Check sheet for the modelled part. Datum: model origin and axes. Units: mm. Face numbers are marked on the shaded views. A direction names the side the tool comes from. Give positions to 0.01 mm unless a question says otherwise; leave off trailing zeros. Order: outer loops, then holes, each group sorted by start corner. A loop starts at its lowest first (then second) coordinate and runs counter-clockwise, first axis right, second up. Notation, with made-up numbers: (-17.5, 37.25) - (27.5, 37.25) arc R22 cw to (27.5, 46.25) - close; hole circle Ø3 at (38, -7.75). An arc over 180 degrees is marked (long way). Answer in a Markdown table with one row per item.
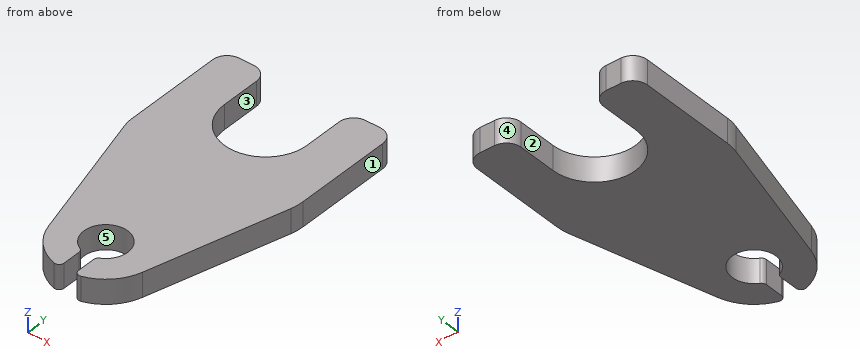
from build123d import *

# Parameters (mm, degrees)
BASE_EXTRUDE_DEPTH = 5


with BuildPart() as part:
    # Sketch1 → Base-Extrude (new body)
    with BuildSketch(Plane.XY):
        with BuildLine():
            Line((1.5, -4.898979486), (1.5, -8.645808233))
            ThreePointArc((1.5, -8.645808233), (1.899074787, -9.445113487), (2.777777778, -9.606453592))
            ThreePointArc((2.777777778, -9.606453592), (7.140306068, -7.001144853), (9.659258263, -2.588190451))
            Line((9.659258263, -2.588190451), (17.159258263, 25.402190606))
            ThreePointArc((17.159258263, 25.402190606), (17.414448614, 26.685119135), (17.5, 27.990381057))
            Line((17.5, 27.990381057), (17.5, 48))
            ThreePointArc((17.5, 48), (16.621320344, 50.121320344), (14.5, 51))
            Line((14.5, 51), (11.5, 51))
            ThreePointArc((11.5, 51), (9.378679656, 50.121320344), (8.5, 48))
            Line((8.5, 48), (8.5, 40))
            ThreePointArc((8.5, 40), (0, 31.5), (-8.5, 40))
            Line((-8.5, 40), (-8.5, 48))
            ThreePointArc((-8.5, 48), (-9.378679656, 50.121320344), (-11.5, 51))
            Line((-11.5, 51), (-14.5, 51))
            ThreePointArc((-14.5, 51), (-16.621320344, 50.121320344), (-17.5, 48))
            Line((-17.5, 48), (-17.5, 27.990381057))
            ThreePointArc((-17.5, 27.990381057), (-17.414448614, 26.685119135), (-17.159258263, 25.402190606))
            Line((-17.159258263, 25.402190606), (-9.659258263, -2.588190451))
            ThreePointArc((-9.659258263, -2.588190451), (-7.140306068, -7.001144853), (-2.777777778, -9.606453592))
            ThreePointArc((-2.777777778, -9.606453592), (-1.899074787, -9.445113487), (-1.5, -8.645808233))
            Line((-1.5, -8.645808233), (-1.5, -4.898979486))
            ThreePointArc((-1.5, -4.898979486), (-1.647197135, -4.376746518), (-2.045454545, -4.008255943))
            ThreePointArc((-2.045454545, -4.008255943), (0, 4.5), (2.045454545, -4.008255943))
            ThreePointArc((2.045454545, -4.008255943), (1.647197135, -4.376746518), (1.5, -4.898979486))
        make_face()
    extrude(amount=BASE_EXTRUDE_DEPTH)


solid = part.part
(1) Thickness scan on L1, parallel to X at y = 45.5, z = 0.9; L2, parallel to X at y = 0, z = 2.25; L3, parallel to Y at x = 4, z = 4.2. Record the ranges inside material, lowest first.
Geometry says:
| item | result |
|---|---|
| L1 | -17.5 to -8.5, 8.5 to 17.5 |
| L2 | -10.35 to -4.5, 4.5 to 10.35 |
| L3 | -9.17 to -2.06, 2.06 to 32.5 |
(2) Cross-section at B-B, the plane z = 2.6. Record the cut outline in (x, y), then the cut area to 3 significant figures.
Geometry says:
| item | result |
|---|---|
| outline | (-17.5, 27.99) arc R10 ccw to (-17.16, 25.4) - (-9.66, -2.59) arc R10 ccw to (-2.78, -9.61) arc R1 ccw to (-1.5, -8.65) - (-1.5, -4.9) arc R1 ccw to (-2.05, -4.01) arc R4.5 cw (long way) to (2.05, -4.01) arc R1 ccw to (1.5, -4.9) - (1.5, -8.65) arc R1 ccw to (2.78, -9.61) arc R10 ccw to (9.66, -2.59) - (17.16, 25.4) arc R10 ccw to (17.5, 27.99) - (17.5, 48) arc R3 ccw to (14.5, 51) - (11.5, 51) arc R3 ccw to (8.5, 48) - (8.5, 40) arc R8.5 cw to (-8.5, 40) - (-8.5, 48) arc R3 ccw to (-11.5, 51) - (-14.5, 51) arc R3 ccw to (-17.5, 48) - close |
| area | 1,360 mm² |
(3) Mould release check, pull along Y, two halves, no side actions. Record for the marked faces 3, 4 and 5: pulls with the +Y half, pulls with the -Y half, needs draft (parallel to the pull), parting line crosses it, or undercut.
Geometry says:
| item | result |
|---|---|
| face 3 | needs draft |
| face 4 | pulls with the +Y half |
| face 5 | undercut |
(4) Cross-section at A-A, the plane y = 42. Record the cut outline in (x, z).
Geometry says:
| item | result |
|---|---|
| outline | (-17.5, 0) - (-8.5, 0) - (-8.5, 5) - (-17.5, 5) - close; (8.5, 0) - (17.5, 0) - (17.5, 5) - (8.5, 5) - close |
(5) Cross-section at D-D, the plane y = 0. Record the cut outline in (x, z), then the cut area to 3 significant figures.
Geometry says:
| item | result |
|---|---|
| outline | (-10.35, 0) - (-4.5, 0) - (-4.5, 5) - (-10.35, 5) - close; (4.5, 0) - (10.35, 0) - (10.35, 5) - (4.5, 5) - close |
| area | 58.5 mm² |
(6) Access from +Z, -Z, +X, -X, +Y, -Y to the whole of each face (thin tool, end or side, straight path). Record for the marked faces 1 and 2.
Geometry says:
| item | result |
|---|---|
| face 1 | +Z, -Z, +X, +Y, -Y |
| face 2 | +Z, -Z, +Y |
(7) Cross-section at C-C, the plane x = 0. Record the cut outline in (y, z).
Geometry says:
| item | result |
|---|---|
| outline | (4.5, 0) - (31.5, 0) - (31.5, 5) - (4.5, 5) - close |
(8) Gauge pin test, flat ends, axial feed: P1, Ø1.9, axis at y = -7.5, z = 2.5, coming from the +X side; P2, Ø1, axis at x = -5.5, z = 3, coming from the -Y side; P3, Ø1.9, axis at y = -6, z = 2.5, coming from the -X side. Record the tip position at first contact, or that the pin passes through.
Geometry says:
| item | result |
|---|---|
| P1 | x = 7.56 |
| P2 | y = -8.66 |
| P3 | x = -8.63 |
